```python
from build123d import *

# Parameters (mm, degrees)
SKETCH1_R           = 6
BOSS_EXTRUDE1_DEPTH = 90
SKETCH2_W           = 25
SKETCH2_H           = 3.681667676
SKETCH3_R           = 7.5
CUT_EXTRUDE1_DEPTH  = 20


with BuildPart() as part:
    # Sketch1 → Boss-Extrude1 (new body)
    with BuildSketch(Plane.XY):
        with Locations(Location((0, 0, 0), (0, 0, 180))):
            Circle(SKETCH1_R)
    extrude(amount=BOSS_EXTRUDE1_DEPTH)

    # Sketch2 → Revolve1 (revolve)
    with BuildSketch(Plane(origin=(0, 0, 0), x_dir=(0, 0, -1), z_dir=(1, 0, 0)), mode=Mode.PRIVATE) as revolve1_sk:
        with Locations((-12.5, 7.840833838)):
            Rectangle(SKETCH2_W, SKETCH2_H)
    revolve(revolve1_sk.sketch.rotate(Axis((0, 0.181667676, 35.200849853), (0, 0, -1)), 90), axis=Axis((0, 0.181667676, 35.200849853), (0, 0, -1)))

    # Sketch3 → Cut-Extrude1 (cut)
    with BuildSketch(Plane(origin=(0, 0, 0), x_dir=(-1, 0, 0), z_dir=(0, 0, -1))):
        Circle(SKETCH3_R)
    extrude(amount=-CUT_EXTRUDE1_DEPTH, mode=Mode.SUBTRACT)


solid = part.part
```
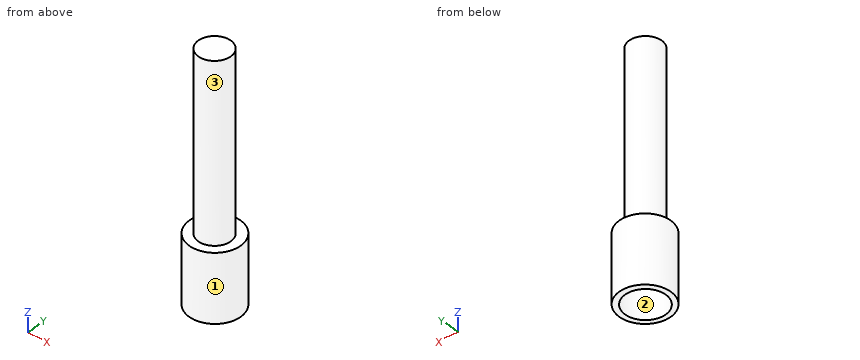
Input: part model. Units: mm. Frame: model coordinates. Face numbers are marked on the shaded views. A direction names the side the tool comes from. Round coordinates to 2 decimals unless told otherwise and drop trailing zeros. Loops run counter-clockwise (first coordinate to the right, second up) from the corner with the lowest first, then second, coordinate; pieces in that order, holes last. Notation, with made-up numbers: M 5,-31 L 32,-31 A30 ccw 32,-2 Z; hole C 71.5,11.5 d8. An arc over 180 degrees is marked long. Answer in a Markdown table with one row per item. Add a question column.
1. Section C-C (z = 11.5). Output: boundary loops of the cut face in (x, y).
2. Contact query for flat-ended pins moving along their axis: pin 1 (2 mm diameter, centred on y = -3.5, z = 59, fed in from +X); pin 2 (2 mm diameter, centred on y = -2, z = 75.5, fed in from -X); pin 3 (5 mm diameter, centred on y = -2.5, z = 70.5, fed in from -X). Output: stop coordinate, or through.
3. Set-up query: the marked faces 1, 2 and 3. Return all of +Z, -Z, +X, -X, +Y, -Y with unobstructed straight access to the full face (end or side cutting, diameter ignored); none if empty.
4. Section A-A (x = 0). Output: boundary loops of the cut face in (y, z), and give its area (3 significant figures).
5. Ray query, probe 1 along Y at (x, z) = (0, 15); probe 2 along Z at (x, y) = (3.5, -0.75); probe 3 along Z at (x, y) = (3, -8). Return the intervals inside material, ascending.
6. Section B-B (y = -5). Output: boundary loops of the cut face in (x, z).
7. Section D-D (z = 23.5). Output: boundary loops of the cut face in (x, y), and give its area (3 significant figures).
Values follow:
| question | item | result |
|---|---|---|
| 1 | outline | C 0,0.18 d19; hole C 0,0 d15 |
| 2 | pin 1 | x = 5.45 |
| 2 | pin 2 | x = -5.92 |
| 2 | pin 3 | x = -6 |
| 3 | face 1 | +Z, -Z |
| 3 | face 2 | -Z |
| 3 | face 3 | +Z |
| 4 | outline | M -9.32,0 L -7.5,0 L -7.5,20 L 7.5,20 L 7.5,0 L 9.68,0 L 9.68,25 L 6,25 L 6,90 L -6,90 L -6,25 L -9.32,25 Z |
| 4 | area | 955 mm^2 |
| 5 | probe 1 | -9.32 to -7.5, 7.5 to 9.68 |
| 5 | probe 2 | 20 to 90 |
| 5 | probe 3 | 0 to 25 |
| 6 | outline | M -7.96,0 L -5.59,0 L -5.59,20 L 5.59,20 L 5.59,0 L 7.96,0 L 7.96,25 L 3.32,25 L 3.32,90 L -3.32,90 L -3.32,25 L -7.96,25 Z |
| 7 | outline | C 0,0.18 d19 |
| 7 | area | 284 mm^2 |
